```python
from build123d import *

# Parameters (mm, degrees)
SKETCH1_W                = 43
SKETCH1_H                = 51
BOSS_EXTRUDE1_DEPTH      = 12
SKETCH2_W                = 7
SKETCH2_H                = 51
BOSS_EXTRUDE2_DEPTH      = 24
BOSS_EXTRUDE2_DEPTH_BACK = 12
SKETCH3_R                = 1.375
SKETCH3_R_2              = 2
CUT_EXTRUDE1_DEPTH       = 12


with BuildPart() as part:
    # Sketch1 → Boss-Extrude1 (new body)
    with BuildSketch(Plane(origin=(0, 0, 0), x_dir=(1, 0, 0), z_dir=(0, 1, 0))):
        Rectangle(SKETCH1_W, SKETCH1_H)
    extrude(amount=BOSS_EXTRUDE1_DEPTH)

    # Sketch2 → Boss-Extrude2 (add, two sides)
    with BuildSketch(Plane(origin=(0, 12, 0), x_dir=(1, 0, 0), z_dir=(0, 1, 0))) as boss_extrude2_sk:
        with Locations((25, 0)):
            Rectangle(SKETCH2_W, SKETCH2_H)
    extrude(amount=BOSS_EXTRUDE2_DEPTH)
    extrude(boss_extrude2_sk.sketch, amount=-BOSS_EXTRUDE2_DEPTH_BACK)

    # Sketch3 → Cut-Extrude1 (cut)
    with BuildSketch(Plane(origin=(0, 12, 0), x_dir=(1, 0, 0), z_dir=(0, 1, 0))):
        with Locations((17.5, 0)):
            Circle(SKETCH3_R)
        with Locations((-17.5, 0)):
            Circle(SKETCH3_R)
        with Locations((13.775, 15.513813063)):
            Circle(SKETCH3_R_2)
        with Locations((-13.775, 15.513813063)):
            Circle(SKETCH3_R_2)
        with Locations((13.775, -13.486186937)):
            Circle(SKETCH3_R_2)
        with Locations((-13.775, -13.486186937)):
            Circle(SKETCH3_R_2)
    extrude(amount=-CUT_EXTRUDE1_DEPTH, mode=Mode.SUBTRACT)


solid = part.part
```
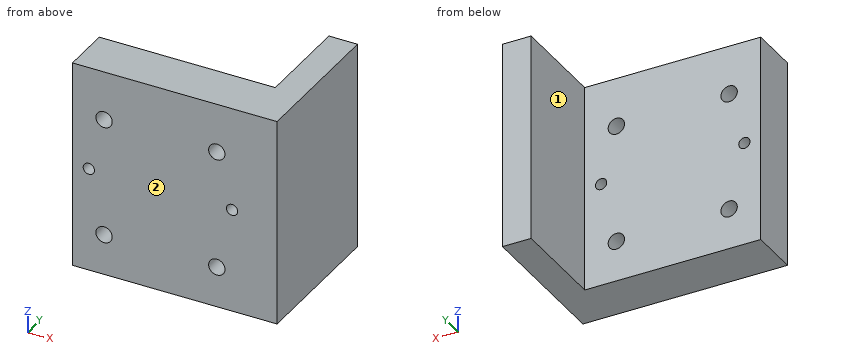
Input: part model. Units: mm. Frame: model coordinates. Face numbers are marked on the shaded views. A direction names the side the tool comes from. Give positions to 0.01 mm unless a question says otherwise; leave off trailing zeros. Loops run counter-clockwise (first coordinate to the right, second up) from the corner with the lowest first, then second, coordinate; pieces in that order, holes last.
1) Section query B-B on x = 17.5. Return the cut outline in (y, z) (3 decimals).
A:
outline: (0, -25.5) - (12, -25.5) - (12, -1.375) - (0, -1.375) - close; (0, 1.375) - (12, 1.375) - (12, 25.5) - (0, 25.5) - close
2) Section query A-A on z = 0. Return the cut outline in (x, y) (3 decimals), and give its area (3 significant figures).
A:
outline: (-21.5, 0) - (-18.875, 0) - (-18.875, 12) - (-21.5, 12) - close; (-16.125, 0) - (16.125, 0) - (16.125, 12) - (-16.125, 12) - close; (18.875, 0) - (28.5, 0) - (28.5, 36) - (21.5, 36) - (21.5, 12) - (18.875, 12) - close
area: 702 mm2
3) Section query C-C on y = 5. Return the cut outline in (x, z) (3 decimals), and give its area (3 significant figures).
A:
outline: (-21.5, -25.5) - (28.5, -25.5) - (28.5, 25.5) - (-21.5, 25.5) - close; hole circle Ø2.75 at (-17.5, 0); hole circle Ø4 at (-13.775, -15.514); hole circle Ø4 at (-13.775, 13.486); hole circle Ø4 at (13.775, -15.514); hole circle Ø4 at (13.775, 13.486); hole circle Ø2.75 at (17.5, 0)
area: 2,490 mm2
4) Reachability of the marked faces 1 and 2 from +Z, -Z, +X, -X, +Y, -Y: full face, straight path, thin tool, end or side. Return the list, or none.
A:
face 1: +Z, -Z, -X, +Y
face 2: +Z, -Z, +X, -X, -Y
5) Contact query for flat-ended pins moving along their axis: pin 1 (3.5 mm diameter, centred on x = -17.5, z = 0, fed in from +Y); pin 2 (7 mm diameter, centred on y = 26.5, z = -0.5, fed in from -X). Output: stop coordinate, or through.
A:
pin 1: stops at y = 12
pin 2: stops at x = 21.5
6) Line query: L1, parallel to X at y = 8.75, z = 0 (3 decimals); L2, parallel to Z at x = 17.5, y = 7.25 (3 decimals); L3, parallel to X at y = 18, z = -20.5. Output: solid intervals per line, ascending.
A:
L1: x = -21.5 to -18.875, -16.125 to 16.125, 18.875 to 28.5
L2: z = -25.5 to -1.375, 1.375 to 25.5
L3: x = 21.5 to 28.5
7) Section query D-D on z = 9.5. Return the cut outline in (x, y), and give its area (3 significant figures).
A:
outline: (-21.5, 0) - (28.5, 0) - (28.5, 36) - (21.5, 36) - (21.5, 12) - (-21.5, 12) - close
area: 768 mm2
